Solid Edge part; units mm, degrees
sketch "Sketch1" plane through (0, 0, 0) normal (0, 0, 1) x (1, 0, 0)
  circle A0 centre (0, 0) radius 1.5
extrude "Protrusion1" add sketch "Sketch1" along normal blind 6.25
sketch "Sketch2" plane through (0, 0, 6.25) normal (0, 0, 1) x (1, 0, 0)
  circle A0 centre (0, 0) radius 3
extrude "ExtrudedProtrusion_2" add sketch "Sketch2" along normal blind 1.75
chamfer "Chamfer_1" distance 1.75 angle 45 1 edges at (-3, 0, 6.25)
sketch "Sketch3" plane through (0, 0, 8) normal (0, 0, 1) x (0, 1, 0)
  line L0 (0.8978, -1.555) -> (1.7956, 0)
  line L1 (1.7956, 0) -> (0.8978, 1.555)
  line L2 (0.8978, 1.555) -> (-0.8978, 1.555)
  line L3 (-0.8978, 1.555) -> (-1.7956, 0)
  line L4 (-1.7956, 0) -> (-0.8978, -1.555)
  line L5 (-0.8978, -1.555) -> (0.8978, -1.555)
extrude "ExtrudedCutout_1" cut sketch "Sketch3" against normal blind 1
properties material "Iron, grey cast type 20"
The model under review builds one solid part; all positions refer to its coordinate system, in mm. A direction names the side the tool comes from. Round coordinates to 2 decimals unless told otherwise and drop trailing zeros. Order: outer loops, then holes, each group sorted by start corner. A loop starts at its lowest first (then second) coordinate and runs counter-clockwise, first axis right, second up.
(1) Tool access review of faces 4 (the face through (0.77, -1.35, 7.51)), 5 (the face through (0, 0, 0)), 6 (the face through (-1.5, -0.07, 3.2)): name each direction out of +Z, -Z, +X, -X, +Y, -Y from which nothing blocks a thin tool from reaching the whole face with its end or side.
Working result:
face 4: +Z
face 5: -Z, +X, -X, +Y, -Y
face 6: -Z
(2) Mouldability with a two-part tool opening along Y and no side actions: class faces 1 (the face through (-0.79, -1.34, 7.51)), 2 (the face through (1.3, -1.3, 8)), 3 (the face through (0, -2, 7)) as released by +Y, released by -Y, zero draft, split by the parting line, or undercut.
Working result:
face 1: undercut
face 2: zero draft
face 3: split by the parting line
(3) Wall thickness on L1, parallel to Z at x = 0.65, y = 1; L2, parallel to Y at x = -0.15, z = 7.25 (3 decimals); L3, parallel to Z at x = -1.2, y = -1.3: over which ranges is each line inside the solid? List them lowest first.
Working result:
L1: z = 0 to 7
L2: y = -2.245 to -1.709, 1.709 to 2.245
L3: z = 6.77 to 8
(4) For P1, Ø2, axis at y = -1, z = 5, coming from the -X side; P2, Ø1, axis at x = 1.5, y = 1.5, coming from the -Z side; P3, Ø1.6, axis at x = -0.5, y = 0, coming from the +Z side, all flat-tipped, find the tip position at first contact; note any pin that passes through.
Working result:
P1: stops at x = -1.5
P2: stops at z = 6.62
P3: stops at z = 7
(5) Take a section at B-B, the plane z = 5.5. State the section outline as (x, y) points.
Working result:
outline: circle Ø3 at (0, 0)
(6) Take a section at A-A, the plane y = 0. State the section outline as (x, z) points (3 decimals), plus the area to 3 significant figures.
Working result:
outline: (-3, 8) - (-1.5, 6.5) - (-1.5, 0) - (1.5, 0) - (1.5, 6.5) - (3, 8) - (1.555, 8) - (1.555, 7) - (-1.555, 7) - (-1.555, 8) - close
area: 23.1 mm2
